from build123d import *

# Parameters (mm, degrees)
F0_W      = 300
F0_H      = 450.8
F0_R      = 1.9
F2_DEPTH  = 5
F1_R      = 0.5
F3_DEPTH  = 25
F4_W      = 147.6
F4_H      = 123.8
F5_DEPTH  = 25
F6_R      = 25
F7_W      = 14
F7_H      = 15.5
F8_DEPTH  = 25
F9_R      = 7.5
F10_DEPTH = 25
F9_R_2    = 2
F11_DEPTH = 25


with BuildPart() as f2:
    # F0 (on Top) → F2 (new body)
    with BuildSketch(Plane.XY):
        Rectangle(F0_W, F0_H)
        with Locations((-132.5, -215.4)):
            Circle(F0_R, mode=Mode.SUBTRACT)
        with Locations((-17.5, -215.4)):
            Circle(F0_R, mode=Mode.SUBTRACT)
        with BuildLine():
            ThreePointArc((19.4, -215.4), (17.5, -217.3), (15.6, -215.4))
            ThreePointArc((15.6, -215.4), (17.5, -213.5), (19.4, -215.4))
        make_face(mode=Mode.SUBTRACT)
        with Locations((132.5, -215.4)):
            Circle(F0_R, mode=Mode.SUBTRACT)
        with Locations((-132.5, 215.4)):
            Circle(F0_R, mode=Mode.SUBTRACT)
        with Locations((-17.5, 215.4)):
            Circle(F0_R, mode=Mode.SUBTRACT)
        with Locations((17.5, 215.4)):
            Circle(F0_R, mode=Mode.SUBTRACT)
        with Locations((132.5, 215.4)):
            Circle(F0_R, mode=Mode.SUBTRACT)
    extrude(amount=-F2_DEPTH)

    # F1 (on Top) → F3 (cut)
    with BuildSketch(Plane.XY):
        with Locations((-105, 202.4)):
            Circle(F1_R)
        with Locations((105, 202.4)):
            Circle(F1_R)
        with Locations((105, -107.6)):
            Circle(F1_R)
        with Locations((-105, -107.6)):
            Circle(F1_R)
    extrude(amount=-F3_DEPTH, mode=Mode.SUBTRACT)

    # F4 (on face) → F5 (cut)
    with BuildSketch(Plane.XY):
        with Locations((0, 112.7)):
            Rectangle(F4_W, F4_H)
        with Locations((0, -112.7)):
            Rectangle(F4_W, F4_H)
    extrude(amount=-F5_DEPTH, mode=Mode.SUBTRACT)

    # F6
    f6_edges = [f2.edges().sort_by_distance(p)[0] for p in [
        (-73.8, 174.6, -2.5),
        (73.8, 174.6, -2.5),
        (-73.8, 50.8, -2.5),
        (73.8, 50.8, -2.5),
        (-73.8, -50.8, -2.5),
        (73.8, -50.8, -2.5),
        (73.8, -174.6, -2.5),
        (-73.8, -174.6, -2.5),
    ]]
    fillet(f6_edges, radius=F6_R)

    # F7 (on face) → F8 (cut)
    with BuildSketch(Plane.XY):
        with Locations((-116, 120.65)):
            Rectangle(F7_W, F7_H)
    extrude(amount=-F8_DEPTH, mode=Mode.SUBTRACT)

    # F9 (on face) → F10 (cut)
    with BuildSketch(Plane.XY):
        with Locations((-115, -130.4)):
            Circle(F9_R)
    extrude(amount=-F10_DEPTH, mode=Mode.SUBTRACT)

    # F9 (on face) → F11 (cut)
    with BuildSketch(Plane.XY):
        with Locations((-107, -10.4)):
            Circle(F9_R_2)
        with Locations((-123, -10.4)):
            Circle(F9_R_2)
    extrude(amount=-F11_DEPTH, mode=Mode.SUBTRACT)


solid = f2.part
Input: part model. Units: mm. Frame: model coordinates. A direction names the side the tool comes from. Give positions to 0.01 mm unless a question says otherwise; leave off trailing zeros. Write each loop counter-clockwise with the first axis right and the second up, starting at its lowest first coordinate (ties: lowest second). Pieces come first, ordered by that corner, then holes. Notation, with made-up numbers: M 31,83 L 87,83 A8 ccw 87,88 Z; hole C 56,-5.5 d4. An arc over 180 degrees is marked long. Use one line per item in the form item = value.
1. Cut plane D-D on y = 154.5. Return loops of the section in (x, z).
Outcome:
outline = M -150,-5 L -73.32,-5 L -73.32,0 L -150,0 Z; M 73.32,-5 L 150,-5 L 150,0 L 73.32,0 Z
2. Cut plane C-C on z = -1.4. State how many separate pieces and enclosed holes the cut face has, and give its area (3 significant figures).
Outcome:
separate_pieces = 1
enclosed_holes = 18
area = 99,300 mm²
3. Reachability of faces 3 (the face through (-2, 3, -5)), 4 (the face through (66.671, -58.318, -2.535)) from +Z, -Z, +X, -X, +Y, -Y: full face, straight path, thin tool, end or side. Return the list, or none.
Outcome:
face_3 = -Z, +X, -X, +Y, -Y
face_4 = +Z, -Z
4. Cut plane B-B on x = -115. Return loops of the section in (y, z).
Outcome:
outline = M -225.4,-5 L -137.9,-5 L -137.9,0 L -225.4,0 Z; M -122.9,-5 L 112.9,-5 L 112.9,0 L -122.9,0 Z; M 128.4,-5 L 225.4,-5 L 225.4,0 L 128.4,0 Z
5. Cut plane A-A on y = -91. Return loops of the section in (x, z), and give its area (3 significant figures).
Outcome:
outline = M -150,-5 L -73.8,-5 L -73.8,0 L -150,0 Z; M 73.8,-5 L 150,-5 L 150,0 L 73.8,0 Z
area = 762 mm²
6. Ray query, L1, parallel to Y at x = 46, z = -2.45; L2, parallel to Y at x = 105, z = -3.6; L3, parallel to Y at x = -17.5, z = -1.5. Return the intervals inside material, ascending.
Outcome:
L1 = -225.4 to -174.6, -50.8 to 50.8, 174.6 to 225.4
L2 = -225.4 to -108.1, -107.1 to 201.9, 202.9 to 225.4
L3 = -225.4 to -217.3, -213.5 to -174.6, -50.8 to 50.8, 174.6 to 213.5, 217.3 to 225.4
7. Mould query, pull axis Y, two halves, no side actions, for faces 1 (the face through (-2, 3, 0)), 2 (the face through (-66.282, -167.471, -2.535)). Classes: released by +Y, released by -Y, zero draft, split by the parting line, or undercut.
Outcome:
face_1 = zero draft
face_2 = undercut
